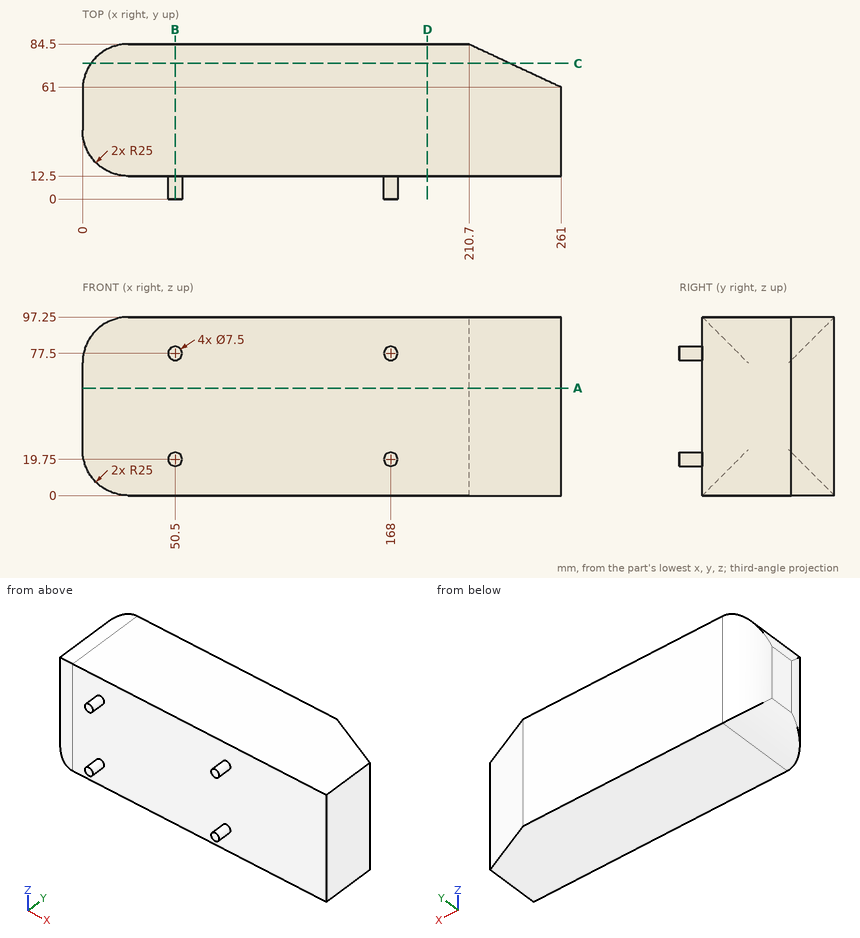
Geometry: see drawing. Coordinates: mm, zero at the bounding-box minimum. Round coordinates to 2 decimals unless told otherwise and drop trailing zeros. Loops run counter-clockwise (first coordinate to the right, second up) from the corner with the lowest first, then second, coordinate; pieces in that order, holes last. Notation, with made-up numbers: (-34, -5) -> (-12, -5) arc R31 ccw to (-12, 23) -> close; hole circle Ø8 at (86, 20.5). An arc over 180 degrees is marked (long way). One line per question, with ' | ' between items. Start each with the question number.
1. Contact query for flat-ended pins moving along their axis: pin 1 (3 mm diameter, centred on x = 226, z = 78, fed in from -Y); pin 2 (6 mm diameter, centred on y = 15.5, z = 61.5, fed in from -X). Output: stop coordinate, or through.
2. Section A-A on z = 58.5. Output: boundary loops of the cut face in (x, y), and give its area (3 significant figures).
3. Line query: line 1 along Y through (x, z) = (198, 79.5); line 2 along X through (y, z) = (42.5, 93.5); line 3 along X through (y, z) = (51, 23). Output: solid intervals per line, ascending. Write a range as [from, to].
4. Section D-D on x = 188. Output: boundary loops of the cut face in (y, z), and give its area (3 significant figures).
5. Section C-C on y = 74. Output: boundary loops of the cut face in (x, z).
6. Section B-B on x = 50.5. Output: boundary loops of the cut face in (y, z), and give its area (3 significant figures).
Returned:
1) pin 1: stops at y = 12.5 | pin 2: stops at x = 8.75
2) outline: (0, 37.5) arc R25 ccw to (25, 12.5) -> (261, 12.5) -> (261, 61) -> (210.7, 84.5) -> (25, 84.5) arc R25 ccw to (0, 59.5) -> close | area: 17,900 mm2
3) line 1: y = [12.5, 84.5] | line 2: x = [11.83, 261] | line 3: x = [0.08, 261]
4) outline: (12.5, 0) -> (84.5, 0) -> (84.5, 97.25) -> (12.5, 97.25) -> close | area: 7,000 mm2
5) outline: (4.63, 10.5) arc R25 ccw to (25, 0) -> (233.17, 0) -> (233.17, 97.25) -> (25, 97.25) arc R25 ccw to (4.63, 86.75) -> close
6) outline: (0, 16) -> (12.5, 16) -> (12.5, 0) -> (84.5, 0) -> (84.5, 97.25) -> (12.5, 97.25) -> (12.5, 81.25) -> (0, 81.25) -> (0, 73.75) -> (12.5, 73.75) -> (12.5, 23.5) -> (0, 23.5) -> close | area: 7,190 mm2
